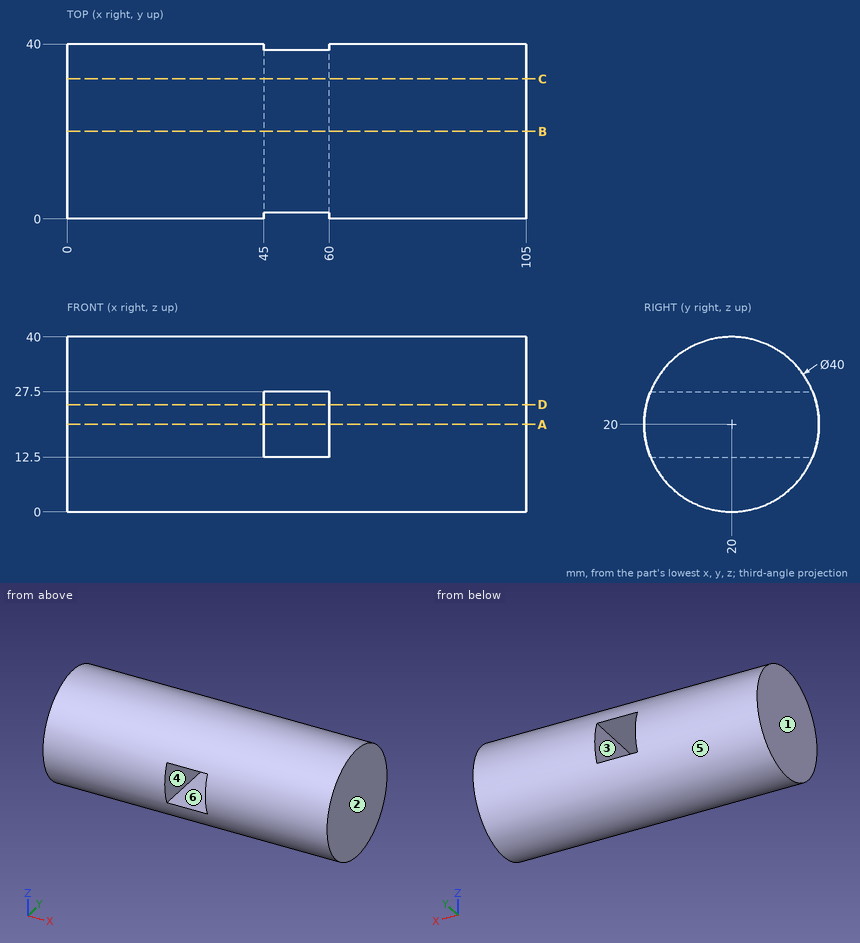
Verification items for this drawing (mm, ordinates from the low corner). A direction names the side the tool comes from. Coordinates: 2 decimals unless noted, no trailing zeros. Loops run counter-clockwise (first coordinate to the right, second up) from the corner with the lowest first, then second, coordinate; pieces in that order, holes last. Notation, with made-up numbers: (62.25, 28.5) -> (91.25, 28.5) arc R35 ccw to (91.25, 66.5) -> close; hole circle Ø3 at (39, -29.75). An arc over 180 degrees is marked (long way). Put each result on its own line as item: value.
1. Gauge pin test, flat ends, axial feed: P1, Ø5, axis at x = 20.5, y = 15, coming from the -Z side; P2, Ø5, axis at x = 92.5, z = 14, coming from the -Y side; P3, Ø6, axis at x = 23.5, z = 32.5, coming from the -Y side. Record the tip position at first contact, or that the pin passes through.
Result set:
P1: stops at z = 0.16
P2: stops at y = 0.31
P3: stops at y = 2.4
2. Section check C-C, the plane y = 32. Record the boundary of the cut face in (x, z), then the cut area to 4 significant figures.
Result set:
outline: (0, 4) -> (105, 4) -> (105, 36) -> (0, 36) -> close; hole (45, 12.5) -> (60, 12.5) -> (60, 27.5) -> (45, 27.5) -> close
area: 3,135 mm^2
3. Section check D-D, the plane z = 24.5. Record the boundary of the cut face in (x, y), then the cut area to 3 significant figures.
Result set:
outline: (0, 0.51) -> (45, 0.51) -> (45, 39.49) -> (0, 39.49) -> close; (60, 0.51) -> (105, 0.51) -> (105, 39.49) -> (60, 39.49) -> close
area: 3,510 mm^2
4. Section check B-B, the plane y = 20. Record the boundary of the cut face in (x, z), then the cut area to 4 significant figures.
Result set:
outline: (0, 0) -> (105, 0) -> (105, 40) -> (0, 40) -> close; hole (45, 12.5) -> (60, 12.5) -> (60, 27.5) -> (45, 27.5) -> close
area: 3,975 mm^2
5. Mould release check, pull along X, two halves, no side actions. Record for the marked faces 1, 2, 3 and 4: pulls with the +X half, pulls with the -X half, needs draft (parallel to the pull), parting line crosses it, or undercut.
Result set:
face 1: pulls with the -X half
face 2: pulls with the +X half
face 3: undercut
face 4: undercut
6. Section check A-A, the plane z = 20. Record the boundary of the cut face in (x, y).
Result set:
outline: (0, 0) -> (45, 0) -> (45, 40) -> (0, 40) -> close; (60, 0) -> (105, 0) -> (105, 40) -> (60, 40) -> close
7. Tool access check on the marked faces 5 and 6. Record the directions out of +Z, -Z, +X, -X, +Y, -Y that give a thin tool (end or side, any length) a straight path to the whole face; none if there is none.
Result set:
face 5: +X, -X
face 6: +Y, -Y
8. Thickness scan on line 1 (X direction, y = 13, z = 15); line 2 (Z direction, x = 52, y = 13) (3 decimals); line 3 (Z direction, x = 18.5, y = 4.5). Record the ranges inside material, lowest first.
Result set:
line 1: x = 0 to 45, 60 to 105
line 2: z = 1.265 to 12.5, 27.5 to 38.735
line 3: z = 7.36 to 32.64
